Geometry check sheet. Reference: the model listing, model coordinates, mm. A direction names the side the tool comes from. Coordinates: 2 decimals unless noted, no trailing zeros. Write each loop counter-clockwise with the first axis right and the second up, starting at its lowest first coordinate (ties: lowest second). Pieces come first, ordered by that corner, then holes. Notation, with made-up numbers: (36.25, 2.5) -> (73.25, 2.5) arc R15 cw to (73.25, 12.5) -> close; hole circle Ø4 at (-16, 44.25). An arc over 180 degrees is marked (long way). Use a Markdown table: item, result.
```python
from build123d import *

# Parameters (mm, degrees)
SKETCH044_R           = 1.5
EXTRUDE033_DEPTH      = 100
SKETCH047_R           = 2.25
EXTRUDE036_DEPTH      = 7.5
SKETCH046_R           = 1
EXTRUDE035_DEPTH      = 2
EXTRUDE034_DEPTH      = 6.5
SKETCH043_R           = 3.75
EXTRUDE032_DEPTH      = 5
EXTRUDE032_DEPTH_BACK = 4.5
FILLET019_R           = 0.5


with BuildPart() as extrude033:
    # Sketch044 → Extrude033 (new body)
    with BuildSketch(Plane.YZ.offset(34.5)):
        with Locations((-7, -18.25)):
            Circle(SKETCH044_R)
        with Locations((7, -18.25)):
            Circle(SKETCH044_R)
    extrude(amount=-EXTRUDE033_DEPTH)


with BuildPart() as extrude036:
    # Sketch047 → Extrude036 (new body)
    with BuildSketch(Plane.XY.offset(-20)):
        with Locations((26.625, 13.5)):
            Circle(SKETCH047_R)
        with Locations((26.625, -13.5)):
            Circle(SKETCH047_R)
    extrude(amount=-EXTRUDE036_DEPTH)


with BuildPart() as extrude036_1:
    # Extrude036 placement: moved
    add(extrude036.part.moved(Location((0, 0, 3))))


with BuildPart() as fusion015:
    # Sketch046 → Extrude035 (new body)
    with BuildSketch(Plane.XY.offset(-20)):
        with Locations((26.625, 13.5)):
            Circle(SKETCH046_R)
        with Locations((26.625, -13.5)):
            Circle(SKETCH046_R)
    extrude(amount=EXTRUDE035_DEPTH)


with BuildPart() as fusion015_1:
    # Extrude035 placement: moved
    add(fusion015.part.moved(Location((0, 0, 3))))

    # Fusion015: union Extrude036
    add(extrude036_1.part)


with BuildPart() as extrude034:
    # Sketch045 → Extrude034 (new body)
    with BuildSketch(Plane(origin=(0, 0, -15), x_dir=(1, 0, 0), z_dir=(0, 0, -1))):
        Polygon((-22.5, 20.399377), (-22.5, -20.399423), (-34.5, -11.996933), (-34.5, 11.996887), align=None)
    extrude(amount=EXTRUDE034_DEPTH)


with BuildPart() as part_mirroring003:
    # Part__Mirroring003: instance of Extrude034
    add(extrude034.part.mirror(Plane(origin=(0, 0, 0), x_dir=(0, -1, 0), z_dir=(1, 0, 0))))


with BuildPart() as boden_tube_bracket_w_deep_fitting:
    # Sketch043 → Extrude032 (new body, two sides)
    with BuildSketch(Plane.XY.offset(-20)) as extrude032_sk:
        with Locations((26.625, 13.5)):
            Circle(SKETCH043_R)
        with Locations((26.625, -13.5)):
            Circle(SKETCH043_R)
    extrude(amount=EXTRUDE032_DEPTH)
    extrude(extrude032_sk.sketch, amount=-EXTRUDE032_DEPTH_BACK)

    # Fillet019
    fillet019_edges = [boden_tube_bracket_w_deep_fitting.edges().sort_by_distance(p)[0] for p in [
        (22.875, -13.5, -24.5),
        (22.875, 13.5, -24.5),
    ]]
    fillet(fillet019_edges, radius=FILLET019_R)

    # Fusion016: union Part__Mirroring003
    add(part_mirroring003.part)

    # Cut013: cut Fusion015
    add(fusion015_1.part, mode=Mode.SUBTRACT)

    # Cut014: cut Extrude033
    add(extrude033.part, mode=Mode.SUBTRACT)


solid = boden_tube_bracket_w_deep_fitting.part
```
Item 1: Thickness scan on L1, parallel to Z at x = 32.75, y = 7; L2, parallel to Y at x = 25.5, z = -18; L3, parallel to Z at x = 28.5, y = 4.5. Record the ranges inside material, lowest first. Write a range as [from, to].
Answer block:
| item | result |
|---|---|
| L1 | z = [-21.5, -19.75], [-16.75, -15] |
| L2 | y = [-18.3, -15.45], [-11.55, -8.48], [-5.52, 5.52], [8.48, 11.55], [15.45, 18.3] |
| L3 | z = [-21.5, -15] |
Item 2: Depth check by flat-ended pin: P1, Ø1.5, axis at x = 28, z = -20.5, coming from the -Y side; P2, Ø1.3, axis at x = 26, y = 13.5, coming from the -Z side; P3, Ø1, axis at y = -14, z = -21.5, coming from the +X side. Enter the tip coordinate at first touch or a pass-through.
Answer block:
| item | result |
|---|---|
| P1 | stops at y = -17.2 |
| P2 | stops at z = -17 |
| P3 | stops at x = 32.35 |
Item 3: Mould release check, pull along X, two halves, no side actions. Record for faces 1 (the flat face through (28, -14, -17)), 2 (the cylindrical face through (28.77, 14.18, -20.7)), 3 (the cylindrical face through (29.158, -16.265, -21.812)), 4 (the flat face through (26, -16, -24.5)): +X half, -X half, draft (parallel to the pull), parting line (faces both ways), or undercut.
Answer block:
| item | result |
|---|---|
| face 1 | undercut |
| face 2 | undercut |
| face 3 | parting line |
| face 4 | draft |
Item 4: Section check D-D on x = 33. Record the boundary of the cut face in (y, z), then the cut area to 3 significant figures.
Answer block:
| item | result |
|---|---|
| outline | (-13.05, -21.5) -> (13.05, -21.5) -> (13.05, -15) -> (-13.05, -15) -> close; hole circle Ø3 at (-7, -18.25); hole circle Ø3 at (7, -18.25) |
| area | 155 mm^2 |
Item 5: Tool access check on faces 5 (the flat face through (28, 0, -15)), 6 (the flat face through (28, 13, -17)). Record the directions out of +Z, -Z, +X, -X, +Y, -Y that give a thin tool (end or side, any length) a straight path to the whole face; none if there is none.
Answer block:
| item | result |
|---|---|
| face 5 | +Z, +X, -X, +Y, -Y |
| face 6 | -Z |
Item 6: Section check A-A on z = -18.25. Record the boundary of the cut face in (x, y) (3 decimals), then the cut area to 3 significant figures.
Answer block:
| item | result |
|---|---|
| outline | (22.5, -20.399) -> (27.029, -17.228) arc R3.75 ccw to (29.99, -15.155) -> (34.5, -11.997) -> (34.5, -8.5) -> (22.5, -8.5) -> close; (22.5, -5.5) -> (34.5, -5.5) -> (34.5, 5.5) -> (22.5, 5.5) -> close; (22.5, 8.5) -> (34.5, 8.5) -> (34.5, 11.997) -> (29.99, 15.155) arc R3.75 ccw to (27.029, 17.228) -> (22.5, 20.399) -> close; hole circle Ø4.5 at (26.625, -13.5); hole circle Ø4.5 at (26.625, 13.5) |
| area | 287 mm^2 |
Item 7: Section check B-B on y = -7. Record the boundary of the cut face in (x, z).
Answer block:
| item | result |
|---|---|
| outline | (22.5, -21.5) -> (34.5, -21.5) -> (34.5, -19.75) -> (22.5, -19.75) -> close; (22.5, -16.75) -> (34.5, -16.75) -> (34.5, -15) -> (22.5, -15) -> close |
Item 8: Section check C-C on z = -20.5. Record the boundary of the cut face in (x, y) (3 decimals), then the cut area to 3 significant figures.
Answer block:
| item | result |
|---|---|
| outline | (22.5, -20.399) -> (27.029, -17.228) arc R3.75 ccw to (29.99, -15.155) -> (34.5, -11.997) -> (34.5, 11.997) -> (29.99, 15.155) arc R3.75 ccw to (27.029, 17.228) -> (22.5, 20.399) -> close; hole circle Ø4.5 at (26.625, -13.5); hole circle Ø4.5 at (26.625, 13.5) |
| area | 359 mm^2 |
